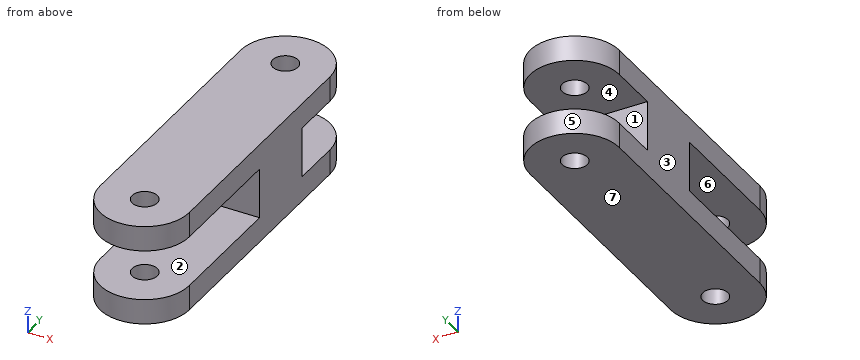
```python
from build123d import *

# Parameters (mm, degrees)
BOSS_EXTRUDE2_DEPTH            = 40
BOSS_EXTRUDE2_DEPTH_BACK       = 40
SKETCH2_R                      = 10
CUT_EXTRUDE1_DEPTH             = 20
CUT_EXTRUDE1_DEPTH_BACK        = 20
CUT_EXTRUDE2_REACH             = 311.987
SKETCH4_W                      = 70.710678118
SKETCH4_H                      = 60
CUT_EXTRUDE2_DIRECTION_2_REACH = 311.987
SHELL1_START                   = -35
SHELL1_OUTLINE_W               = 60.710678118
SHELL1_OUTLINE_H               = 50
SHELL1_DEPTH                   = 70
SHELL1_2_OUTLINE_R             = 15
SHELL1_2_DEPTH                 = 10
SHELL1_START_2                 = 25
SHELL1_3_OUTLINE_R             = 15
SHELL1_3_DEPTH                 = 10


# Read off the part's stored shape, not the designer's step: Shell1
with BuildPart() as part:
    # Sketch2 → Boss-Extrude2 (new, two sides: drawn at the far end of the back side and taken through both)
    with BuildSketch(Plane.XY.offset(-BOSS_EXTRUDE2_DEPTH_BACK)):
        with BuildLine():
            Line((-35.355339059, -70), (-35.355339059, -270))
            ThreePointArc((-35.355339059, -270), (0, -305.355339059), (35.355339059, -270))
            Line((35.355339059, -270), (35.355339059, -70))
            ThreePointArc((35.355339059, -70), (0, -34.644660941), (-35.355339059, -70))
        make_face()
        with Locations((0, -70)):
            Circle(SKETCH2_R, mode=Mode.SUBTRACT)
        with Locations((0, -270)):
            Circle(SKETCH2_R, mode=Mode.SUBTRACT)
    extrude(amount=BOSS_EXTRUDE2_DEPTH + BOSS_EXTRUDE2_DEPTH_BACK)

    # Sketch3 → Cut-Extrude1 (cut, two sides: drawn at the far end of the back side and taken through both)
    with BuildSketch(Plane.XY.offset(-CUT_EXTRUDE1_DEPTH_BACK)):
        with BuildLine():
            Line((-35.355339059, -230), (35.355339059, -230))
            Line((35.355339059, -230), (35.355339059, -270))
            ThreePointArc((35.355339059, -270), (0, -305.355339059), (-35.355339059, -270))
            Line((-35.355339059, -270), (-35.355339059, -230))
        make_face()
        with BuildLine():
            Line((35.355339059, -110), (35.355339059, -70))
            ThreePointArc((35.355339059, -70), (0, -34.644660941), (-35.355339059, -70))
            Line((-35.355339059, -70), (-35.355339059, -110))
            Line((-35.355339059, -110), (35.355339059, -110))
        make_face()
    extrude(amount=CUT_EXTRUDE1_DEPTH + CUT_EXTRUDE1_DEPTH_BACK, mode=Mode.SUBTRACT)

    # Cut-Extrude2: up to this face of the body (flat: up to its plane)
    cut_extrude2_end = Plane(part.part.faces().sort_by_distance((-34.321974306, -250, -20))[0])
    # Sketch4 → Cut-Extrude2 (cut, up to the picked face)
    with BuildSketch(Plane.XY, mode=Mode.PRIVATE) as cut_extrude2_sk1:
        with Locations((0, -200)):
            Rectangle(SKETCH4_W, SKETCH4_H)
    cut_extrude2_tool1 = split(extrude(cut_extrude2_sk1.sketch, amount=-CUT_EXTRUDE2_REACH, mode=Mode.PRIVATE), bisect_by=cut_extrude2_end, keep=Keep.BOTH, mode=Mode.PRIVATE)
    add(cut_extrude2_tool1.solids().sort_by(Axis((0, -200, 0), (0, 0, -1)))[0], mode=Mode.SUBTRACT)

    # Cut-Extrude2 direction 2: up to this face of the body (flat: up to its plane)
    cut_extrude2_direction_2_end = Plane(part.part.faces().sort_by_distance((-34.321974306, -250, 20))[0])
    # Sketch4 → Cut-Extrude2 direction 2 (cut, up to the picked face)
    with BuildSketch(Plane.XY, mode=Mode.PRIVATE) as cut_extrude2_direction_2_sk1:
        with Locations((0, -200)):
            Rectangle(SKETCH4_W, SKETCH4_H)
    cut_extrude2_direction_2_tool1 = split(extrude(cut_extrude2_direction_2_sk1.sketch, amount=CUT_EXTRUDE2_DIRECTION_2_REACH, mode=Mode.PRIVATE), bisect_by=cut_extrude2_direction_2_end, keep=Keep.BOTH, mode=Mode.PRIVATE)
    add(cut_extrude2_direction_2_tool1.solids().sort_by(Axis((0, -200, 0), (0, 0, 1)))[0], mode=Mode.SUBTRACT)

    # Shell1 outline → Shell1 (cut)
    with BuildSketch(Plane.XY.offset(SHELL1_START)):
        with Locations((0, -140)):
            Rectangle(SHELL1_OUTLINE_W, SHELL1_OUTLINE_H)
    extrude(amount=SHELL1_DEPTH, mode=Mode.SUBTRACT)

    # Shell1 2 outline → Shell1 2 (cut)
    # profile 1 of 2: a face of its own
    with BuildSketch(Plane.XY.offset(SHELL1_START)):
        with BuildLine():
            ThreePointArc((-30.355339059, -270), (0, -300.355339059), (30.355339059, -270))
            Line((30.355339059, -270), (30.355339059, -165))
            Line((30.355339059, -165), (-30.355339059, -165))
            Line((-30.355339059, -165), (-30.355339059, -270))
        make_face()
        with Locations((0, -270)):
            Circle(SHELL1_2_OUTLINE_R, mode=Mode.SUBTRACT)
    # profile 2 of 2: a face of its own
    with BuildSketch(Plane.XY.offset(SHELL1_START)):
        with BuildLine():
            Line((-30.355339059, -115), (30.355339059, -115))
            Line((30.355339059, -115), (30.355339059, -70))
            ThreePointArc((30.355339059, -70), (0, -39.644660941), (-30.355339059, -70))
            Line((-30.355339059, -70), (-30.355339059, -115))
        make_face()
        with Locations((0, -70)):
            Circle(SHELL1_2_OUTLINE_R, mode=Mode.SUBTRACT)
    extrude(amount=SHELL1_2_DEPTH, mode=Mode.SUBTRACT)

    # Shell1 3 outline → Shell1 3 (cut)
    # profile 1 of 2: a face of its own
    with BuildSketch(Plane.XY.offset(SHELL1_START_2)):
        with BuildLine():
            ThreePointArc((-30.355339059, -270), (0, -300.355339059), (30.355339059, -270))
            Line((30.355339059, -270), (30.355339059, -165))
            Line((30.355339059, -165), (-30.355339059, -165))
            Line((-30.355339059, -165), (-30.355339059, -270))
        make_face()
        with Locations((0, -270)):
            Circle(SHELL1_3_OUTLINE_R, mode=Mode.SUBTRACT)
    # profile 2 of 2: a face of its own
    with BuildSketch(Plane.XY.offset(SHELL1_START_2)):
        with BuildLine():
            Line((-30.355339059, -115), (30.355339059, -115))
            Line((30.355339059, -115), (30.355339059, -70))
            ThreePointArc((30.355339059, -70), (0, -39.644660941), (-30.355339059, -70))
            Line((-30.355339059, -70), (-30.355339059, -115))
        make_face()
        with Locations((0, -70)):
            Circle(SHELL1_3_OUTLINE_R, mode=Mode.SUBTRACT)
    extrude(amount=SHELL1_3_DEPTH, mode=Mode.SUBTRACT)


solid = part.part
```
Can you work these out from the model? Positions are in its coordinate system, mm. Face numbers are marked on the shaded views. A direction names the side the tool comes from. Coordinates: 2 decimals unless noted, no trailing zeros. Loops run counter-clockwise (first coordinate to the right, second up) from the corner with the lowest first, then second, coordinate; pieces in that order, holes last. Notation, with made-up numbers: (5.25, -12) - (55.25, -12) arc R19 cw to (55.25, -1) - close; hole circle Ø3 at (13.25, 13). An arc over 180 degrees is marked (long way). Use a Markdown table: item, result.
Item 1: For the marked faces 1, 2 and 3, which set-ups out of +Z, -Z, +X, -X, +Y, -Y let a thin tool reach every point of the face, with its end or its side?
Numbers:
| item | result |
|---|---|
| face 1 | +X, -X, +Y |
| face 2 | +X, -X, -Y |
| face 3 | +Z, -Z, -X, +Y, -Y |
Item 2: Will these pins go through, and if not, where does the flat tip stop? pin 1 (6 mm diameter, centred on x = 1.5, z = -7, fed in from +Y); pin 2 (12 mm diameter, centred on y = -187, z = 13, fed in from +X); pin 3 (4 mm diameter, centred on x = -25, z = -23, fed in from +Y).
Numbers:
| item | result |
|---|---|
| pin 1 | stops at y = -110 |
| pin 2 | passes through |
| pin 3 | stops at y = -43.15 |
Item 3: I want a section at B-B on z = 32.5. Please give me the cut outline in (x, y), and give its area (3 significant figures).
Numbers:
| item | result |
|---|---|
| outline | (-35.36, -270) arc R35.36 ccw to (35.36, -270) - (35.36, -70) arc R35.36 ccw to (-35.36, -70) - close; circle Ø30 at (0, -270); circle Ø30 at (0, -70); hole (-30.36, -270) arc R30.36 ccw to (30.36, -270) - (30.36, -70) arc R30.36 ccw to (-30.36, -70) - close; hole circle Ø20 at (0, -270); hole circle Ø20 at (0, -70) |
| area | 3,820 mm2 |
Item 4: I want a section at D-D on x = 25.5. Please give me the cut outline in (y, z), and give its area (3 significant figures).
Numbers:
| item | result |
|---|---|
| outline | (-294.49, -40) - (-45.51, -40) - (-45.51, -20) - (-110, -20) - (-110, 20) - (-45.51, 20) - (-45.51, 40) - (-294.49, 40) - (-294.49, 20) - (-170, 20) - (-170, -20) - (-294.49, -20) - close; hole (-286.47, -35) - (-53.53, -35) - (-53.53, -25) - (-115, -25) - (-115, 25) - (-53.53, 25) - (-53.53, 35) - (-286.47, 35) - (-286.47, 25) - (-165, 25) - (-165, -25) - (-286.47, -25) - close |
| area | 5,200 mm2 |
Item 5: I want a section at C-C on z = -13. Please give me the cut outline in (x, y).
Numbers:
| item | result |
|---|---|
| outline | (-35.36, -170) - (35.36, -170) - (35.36, -110) - (-35.36, -110) - close; hole (-30.36, -165) - (30.36, -165) - (30.36, -115) - (-30.36, -115) - close |
Item 6: If I drill on probe 1 along Z at (x, y) = (-6, -207); probe 2 along Y at (x, z) = (0, 29.25); probe 3 along Z at (x, y) = (5, -129.5), over which ranges is the centre line in solid material (lowest first)? Write a range as from..to.
Numbers:
| item | result |
|---|---|
| probe 1 | z = -40..-35, -25..-20, 20..25, 35..40 |
| probe 2 | y = -305.36..-300.36, -285..-280, -260..-255, -85..-80, -60..-55, -39.64..-34.64 |
| probe 3 | z = -40..-35, 35..40 |
Item 7: I want a section at A-A on y = -197. Please give me the cut outline in (x, z).
Numbers:
| item | result |
|---|---|
| outline | (-35.36, -40) - (35.36, -40) - (35.36, -20) - (-35.36, -20) - close; (-35.36, 20) - (35.36, 20) - (35.36, 40) - (-35.36, 40) - close; hole (-30.36, -35) - (30.36, -35) - (30.36, -25) - (-30.36, -25) - close; hole (-30.36, 25) - (30.36, 25) - (30.36, 35) - (-30.36, 35) - close |
Item 8: We'd pull the mould along Z, two halves only. Please class the marked faces 4, 5, 6 and 7: released by +Z, released by -Z, zero draft, split by the parting line, or undercut.
Numbers:
| item | result |
|---|---|
| face 4 | undercut |
| face 5 | zero draft |
| face 6 | undercut |
| face 7 | released by -Z |
